Here's how the part is built. I have some questions about the finished solid (model axes, mm). A direction names the side the tool comes from. Coordinates: 2 decimals unless noted, no trailing zeros. Write each loop counter-clockwise with the first axis right and the second up, starting at its lowest first coordinate (ties: lowest second). Pieces come first, ordered by that corner, then holes.
Item 1: For faces 5 (the face through (4, 0, 4)), 6 (the face through (20.881, 16.052, 6.535)), 7 (the face through (30, -6, 5)), which set-ups out of +Z, -Z, +X, -X, +Y, -Y let a thin tool reach every point of the face, with its end or its side?
Item 2: I want a section at B-B (x = 25). Please give me the cut outline in (y, z).
Item 3: Please list where these lines run through material, in increasing order: line 1 (Y direction, x = 25, z = 3.2); line 2 (Y direction, x = 26.5, z = 2.25); line 3 (Y direction, x = 41.5, z = 7).
Item 4: I want a section at A-A (z = 6.75). Please give me the cut outline in (x, y).
Item 5: If we mould it in two halves opening along Y, with no side actions, what happens to faces 1 (the face through (48, 59, 5)), 2 (the face through (46, 0, 4)), 3 (the face through (30.1, 0.04, 4.44)), 4 (the face through (0, 27, 4))? For each: pulls with the +Y half, pulls with the -Y half, needs draft (parallel to the pull), parting line crosses it, or undercut.
Item 6: I want a section at D-D (z = 2.5). Please give me the cut outline in (x, y), and give its area (3 significant figures).
Item 7: I'm going to push flat-ended pins straight in: P1, Ø5, axis at y = -5, z = 5.5, coming from the -X side; P2, Ø2.5, axis at x = 3.5, z = 4.5, coming from the -Y side; P3, Ø3, axis at x = 15.47, y = 40.1, coming from the -Z side; P4, Ø5, axis at y = -5, z = 3, coming from the +X side. Where does each tip first touch, or does it pass through?
Item 8: I want a section at C-C (y = 40.1). Please give me the cut outline in (x, z).
from build123d import *

# Parameters (mm, degrees)
ESQUISSE1_W                  = 50
ESQUISSE1_H                  = 60
BOSS_EXTRU_1_DEPTH           = 9
ESQUISSE2_W                  = 10
ESQUISSE2_H                  = 9
BOSS_EXTRU_2_DEPTH           = 9
ESQUISSE3_R                  = 8.75
ESQUISSE3_R_2                = 1.65
ENL_V_MAT_EXTRU_1_DEPTH      = 9
ESQUISSE4_R                  = 19
ENL_V_MAT_EXTRU_2_DEPTH      = 5
CONG_1_R                     = 5
ENL_V_MAT_EXTRU_3_DEPTH      = 79.619336044
ENL_V_MAT_EXTRU_3_DEPTH_BACK = 79.619336044


with BuildPart() as part:
    # Esquisse1 → Boss.-Extru.1 (new body)
    with BuildSketch(Plane.XY):
        with Locations((25, 30)):
            Rectangle(ESQUISSE1_W, ESQUISSE1_H)
    extrude(amount=BOSS_EXTRU_1_DEPTH)

    # Esquisse2 → Boss.-Extru.2 (add)
    with BuildSketch(Plane.XY.offset(9)):
        with Locations((35, -4.5)):
            Rectangle(ESQUISSE2_W, ESQUISSE2_H)
        with Locations((15, -4.5)):
            Rectangle(ESQUISSE2_W, ESQUISSE2_H)
    extrude(amount=-BOSS_EXTRU_2_DEPTH)

    # Esquisse3 → Enlèv. mat.-Extru.1 (cut)
    with BuildSketch(Plane.XY.offset(9)):
        with Locations((25, 34.6)):
            Circle(ESQUISSE3_R)
        with Locations((25, 45.6)):
            Circle(ESQUISSE3_R_2)
        with Locations((34.526279442, 40.1)):
            Circle(ESQUISSE3_R_2)
        with Locations((34.526279442, 29.1)):
            Circle(ESQUISSE3_R_2)
        with Locations((25, 23.6)):
            Circle(ESQUISSE3_R_2)
        with Locations((15.473720558, 29.1)):
            Circle(ESQUISSE3_R_2)
        with Locations((15.473720558, 40.1)):
            Circle(ESQUISSE3_R_2)
    extrude(amount=-ENL_V_MAT_EXTRU_1_DEPTH, mode=Mode.SUBTRACT)

    # Esquisse4 → Enlèv. mat.-Extru.2 (cut)
    with BuildSketch(Plane.XY.offset(9)):
        with Locations((25, 34.6)):
            Circle(ESQUISSE4_R)
    extrude(amount=-ENL_V_MAT_EXTRU_2_DEPTH, mode=Mode.SUBTRACT)

    # Congé1
    cong_1_edges = [part.edges().sort_by_distance(p)[0] for p in [
        (0, 60, 4.5),
        (50, 60, 4.5),
    ]]
    fillet(cong_1_edges, radius=CONG_1_R)

    # Esquisse5 → Enlèv. mat.-Extru.3 (cut, two sides: drawn at the far end of the back side and taken through both)
    with BuildSketch(Plane.XY.offset(9).offset(-ENL_V_MAT_EXTRU_3_DEPTH_BACK)):
        with BuildLine():
            Line((27.525126266, 0), (30, -2.474873734))
            ThreePointArc((30, -2.474873734), (30.070710678, 0.070710678), (27.525126266, 0))
        make_face()
        with BuildLine():
            Line((22.474873734, 0), (20, -2.474873734))
            ThreePointArc((20, -2.474873734), (19.929289322, 0.070710678), (22.474873734, 0))
        make_face()
        with BuildLine():
            Line((42.474873734, 0), (40, -2.474873734))
            ThreePointArc((40, -2.474873734), (39.929289322, 0.070710678), (42.474873734, 0))
        make_face()
        with BuildLine():
            Line((7.525126266, 0), (10, -2.474873734))
            ThreePointArc((10, -2.474873734), (10.070710678, 0.070710678), (7.525126266, 0))
        make_face()
    extrude(amount=ENL_V_MAT_EXTRU_3_DEPTH + ENL_V_MAT_EXTRU_3_DEPTH_BACK, mode=Mode.SUBTRACT)


solid = part.part
Answer:
1. face 5: +Z, -Z, -X, -Y
1. face 6: +Z
1. face 7: +Z, -Z, -Y
2. outline: (0, 0) - (21.95, 0) - (21.95, 4) - (15.6, 4) - (15.6, 9) - (0, 9) - close; (25.25, 0) - (25.85, 0) - (25.85, 4) - (25.25, 4) - close; (43.35, 0) - (43.95, 0) - (43.95, 4) - (43.35, 4) - close; (47.25, 0) - (60, 0) - (60, 9) - (53.6, 9) - (53.6, 4) - (47.25, 4) - close
3. line 1: y = 0 to 21.95, 25.25 to 25.85, 43.35 to 43.95, 47.25 to 60
3. line 2: y = 0 to 22.91, 24.29 to 25.98, 43.22 to 44.91, 46.29 to 60
3. line 3: y = 0.55 to 25.18, 44.02 to 60
4. outline: (0, 0) - (7.53, 0) arc R1.75 cw (long way) to (10, -2.47) - (10, -9) - (20, -9) - (20, -2.47) arc R1.75 cw (long way) to (22.47, 0) - (27.53, 0) arc R1.75 cw (long way) to (30, -2.47) - (30, -9) - (40, -9) - (40, -2.47) arc R1.75 cw (long way) to (42.47, 0) - (50, 0) - (50, 55) arc R5 ccw to (45, 60) - (5, 60) arc R5 ccw to (0, 55) - close; hole circle Ø38 at (25, 34.6)
5. face 1: pulls with the +Y half
5. face 2: pulls with the -Y half
5. face 3: undercut
5. face 4: needs draft
6. outline: (0, 0) - (7.53, 0) arc R1.75 cw (long way) to (10, -2.47) - (10, -9) - (20, -9) - (20, -2.47) arc R1.75 cw (long way) to (22.47, 0) - (27.53, 0) arc R1.75 cw (long way) to (30, -2.47) - (30, -9) - (40, -9) - (40, -2.47) arc R1.75 cw (long way) to (42.47, 0) - (50, 0) - (50, 55) arc R5 ccw to (45, 60) - (5, 60) arc R5 ccw to (0, 55) - close; hole circle Ø3.3 at (15.47, 29.1); hole circle Ø3.3 at (15.47, 40.1); hole circle Ø17.5 at (25, 34.6); hole circle Ø3.3 at (25, 23.6); hole circle Ø3.3 at (25, 45.6); hole circle Ø3.3 at (34.53, 29.1); hole circle Ø3.3 at (34.53, 40.1)
6. area: 2,870 mm2
7. P1: stops at x = 10
7. P2: stops at y = 0
7. P3: passes through
7. P4: stops at x = 40
8. outline: (0, 0) - (13.82, 0) - (13.82, 4) - (6.81, 4) - (6.81, 9) - (0, 9) - close; (17.12, 0) - (18.19, 0) - (18.19, 4) - (17.12, 4) - close; (31.81, 0) - (32.88, 0) - (32.88, 4) - (31.81, 4) - close; (36.18, 0) - (50, 0) - (50, 9) - (43.19, 9) - (43.19, 4) - (36.18, 4) - close
